Build history of the part. All positions in model axes, mm. A direction names the side the tool comes from. Round coordinates to 2 decimals unless told otherwise and drop trailing zeros. Order: outer loops, then holes, each group sorted by start corner. A loop starts at its lowest first (then second) coordinate and runs counter-clockwise, first axis right, second up. Notation, with made-up numbers: (-5, -33) -> (39, -33) arc R22 ccw to (39, -7) -> close; hole circle Ø1 at (-27, 86.5). An arc over 180 degrees is marked (long way). Write item = value, one per line.
from build123d import *

# Parameters (mm, degrees)
F0_W     = 50.8
F0_H     = 6.35
F0_R     = 1.143
F0_R_2   = 1.397
F0_R_3   = 1.651
F1_DEPTH = 19.05
F2_R     = 1.27
F4_R     = 3.302
F5_DEPTH = 1.5875


with BuildPart() as f1:
    # F0 (on Top) → F1 (new body)
    with BuildSketch(Plane.XY):
        Rectangle(F0_W, F0_H)
        with Locations((-21.107789129, 0)):
            Circle(F0_R, mode=Mode.SUBTRACT)
        with Locations((-11.3432221115, 0)):
            Circle(F0_R, mode=Mode.SUBTRACT)
        Circle(F0_R_2, mode=Mode.SUBTRACT)
        with Locations((9.8313204944, 0)):
            Circle(F0_R_3, mode=Mode.SUBTRACT)
        with Locations((19.9195742607, 0)):
            Circle(F0_R_3, mode=Mode.SUBTRACT)
    extrude(amount=F1_DEPTH)

    # F2
    f2_edges = [f1.edges().sort_by_distance(p)[0] for p in [
        (0, -3.175, 19.05),
        (0, 3.175, 19.05),
        (-25.4, 0, 19.05),
        (25.4, 0, 19.05),
        (-25.4, -3.175, 9.525),
        (-25.4, 3.175, 9.525),
        (25.4, -3.175, 9.525),
        (25.4, 3.175, 9.525),
        (0, -3.175, 0),
        (0, 3.175, 0),
        (25.4, 0, 0),
        (-25.4, 0, 0),
    ]]
    fillet(f2_edges, radius=F2_R)

    # F4 (on offset) → F5 (cut)
    with BuildSketch(Plane.XZ.offset(3.175)):
        with Locations((13.6511175489, 9.8055116832)):
            Circle(F4_R)
        with Locations((-13.3547777533, 9.8055116832)):
            Circle(F4_R)
    extrude(amount=-F5_DEPTH, mode=Mode.SUBTRACT)


solid = f1.part
Q1. Cut at A-A, the plane y = 0. List the corners of the cut face in (x, z).
Check values:
outline = (-25.4, 1.27) arc R1.27 ccw to (-24.13, 0) -> (-22.25, 0) -> (-22.25, 19.05) -> (-24.13, 19.05) arc R1.27 ccw to (-25.4, 17.78) -> close; (-19.96, 0) -> (-12.49, 0) -> (-12.49, 19.05) -> (-19.96, 19.05) -> close; (-10.2, 0) -> (-1.4, 0) -> (-1.4, 19.05) -> (-10.2, 19.05) -> close; (1.4, 0) -> (8.18, 0) -> (8.18, 19.05) -> (1.4, 19.05) -> close; (11.48, 0) -> (18.27, 0) -> (18.27, 19.05) -> (11.48, 19.05) -> close; (21.57, 0) -> (24.13, 0) arc R1.27 ccw to (25.4, 1.27) -> (25.4, 17.78) arc R1.27 ccw to (24.13, 19.05) -> (21.57, 19.05) -> close
Q2. Cut at B-B, the plane z = 2. List the corners of the cut face in (x, y) (3 decimals), and give its area (3 significant figures).
Check values:
outline = (-25.4, -1.905) arc R1.27 ccw to (-24.13, -3.175) -> (24.13, -3.175) arc R1.27 ccw to (25.4, -1.905) -> (25.4, 1.905) arc R1.27 ccw to (24.13, 3.175) -> (-24.13, 3.175) arc R1.27 ccw to (-25.4, 1.905) -> close; hole circle Ø2.286 at (-21.108, 0); hole circle Ø2.286 at (-11.343, 0); hole circle Ø2.794 at (0, 0); hole circle Ø3.302 at (9.831, 0); hole circle Ø3.302 at (19.92, 0)
area = 290 mm²
Q3. Cut at D-D, the plane z = 10.75. List the corners of the cut face in (x, y) (1 decimal).
Check values:
outline = (-25.4, -1.9) arc R1.3 ccw to (-24.1, -3.2) -> (-16.5, -3.2) -> (-16.5, -1.6) -> (-10.2, -1.6) -> (-10.2, -3.2) -> (10.5, -3.2) -> (10.5, -1.6) -> (16.8, -1.6) -> (16.8, -3.2) -> (24.1, -3.2) arc R1.3 ccw to (25.4, -1.9) -> (25.4, 1.9) arc R1.3 ccw to (24.1, 3.2) -> (-24.1, 3.2) arc R1.3 ccw to (-25.4, 1.9) -> close; hole circle Ø2.3 at (-21.1, 0); hole circle Ø2.3 at (-11.3, 0); hole circle Ø2.8 at (0, 0); hole circle Ø3.3 at (9.8, 0); hole circle Ø3.3 at (19.9, 0)
Q4. Cut at C-C, the plane x = 0. List the corners of the cut face in (y, z) (3 decimals).
Check values:
outline = (-3.175, 1.27) arc R1.27 ccw to (-1.905, 0) -> (-1.397, 0) -> (-1.397, 19.05) -> (-1.905, 19.05) arc R1.27 ccw to (-3.175, 17.78) -> close; (1.397, 0) -> (1.905, 0) arc R1.27 ccw to (3.175, 1.27) -> (3.175, 17.78) arc R1.27 ccw to (1.905, 19.05) -> (1.397, 19.05) -> close
Q5. Probe probe 1 along Y at (x, z) = (0, 4) (3 decimals); probe 2 along X at (y, z) = (1, 2.5); probe 3 along X at (y, z) = (-0.75, 8.25). List the from-to ranges inside material, lowest first.
Check values:
probe_1 = -3.175 to -1.397, 1.397 to 3.175
probe_2 = -25.4 to -21.66, -20.55 to -11.9, -10.79 to -0.98, 0.98 to 8.52, 11.15 to 18.61, 21.23 to 25.4
probe_3 = -25.4 to -21.97, -20.25 to -12.21, -10.48 to -1.18, 1.18 to 8.36, 11.3 to 18.45, 21.39 to 25.4
Q6. Mould opens along Z. For faces 1 (the face through (14, -1.588, 10)), 2 (the face through (0.34, 2.81, 0.38)), 3 (the face through (-22.25, 0.05, 9.39)) say: released by +Z, released by -Z, zero draft, split by the parting line, or undercut.
Check values:
face_1 = undercut
face_2 = released by -Z
face_3 = zero draft
Q7. Which spindle directions (+Z, -Z, +X, -X, +Y, -Y) get a long thin tool onto all of the face, cutting with end or side? Do faces 4 (the face through (-13.78, -2.39, 13.08)), 5 (the face through (25.038, 0.027, 0.382)). Say none if no direction does.
Check values:
face_4 = -Y
face_5 = -Z, +X, +Y, -Y
Q8. Flat gauge pin, fed straight in: pin 1 (3.5 mm diameter, centred on x = -12.5, z = 10.5, fed in from -Y). Where does the tip first touch, or does it go through?
Check values:
pin_1 = -1.59
